from build123d import *

# Parameters (mm, degrees)
SKETCH1_W                  = 177.8
SKETCH1_H                  = 25.4
BOSS_EXTRUDE1_DEPTH        = 9.525
F_1_2_0_5_DIAMETER_HOLE1_D = 12.7
SKETCH6_W                  = 17.78
SKETCH6_H                  = 25.4
CUT_EXTRUDE2_DEPTH         = 180.857514786


with BuildPart() as part:
    # Sketch1 → Boss-Extrude1 (new body)
    with BuildSketch(Plane.XY):
        with Locations((88.9, 12.7)):
            Rectangle(SKETCH1_W, SKETCH1_H)
    extrude(amount=BOSS_EXTRUDE1_DEPTH)

    # 1/2 (0.5) Diameter Hole1 (through all)
    with Locations(Plane.XY.offset(9.525)):
        with Locations((12.7, 12.7), (147.32, 12.7)):
            Hole(F_1_2_0_5_DIAMETER_HOLE1_D / 2)

    # Sketch6 → Cut-Extrude2 (cut, through all)
    with BuildSketch(Plane.XY.offset(9.525)):
        with Locations((168.91, 12.7)):
            Rectangle(SKETCH6_W, SKETCH6_H)
    extrude(amount=-CUT_EXTRUDE2_DEPTH, mode=Mode.SUBTRACT)


solid = part.part
The listing builds one solid part. Answer for the finished solid, in the listing's coordinates (mm). Give positions to 0.01 mm unless a question says otherwise; leave off trailing zeros. Loops run counter-clockwise (first coordinate to the right, second up) from the corner with the lowest first, then second, coordinate; pieces in that order, holes last. Notation, with made-up numbers: (52, 13) - (70, 13) arc R34 ccw to (70, 45) - close; hole circle Ø9 at (87, 18). An arc over 180 degrees is marked (long way). Write each question's results on one line, items separated by ' | '.
1. A flat-ended cylindrical pin translates along its axis: P1, Ø3, axis at x = 72, z = 2.5, coming from the -Y side. Find the tip coordinate at first contact, or state that the pin passes through.
Resolved:
P1: stops at y = 0
2. Find section C-C, the plane z = 1.5. Write down the section's boundary in (x, y).
Resolved:
outline: (0, 0) - (160.02, 0) - (160.02, 25.4) - (0, 25.4) - close; hole circle Ø12.7 at (12.7, 12.7); hole circle Ø12.7 at (147.32, 12.7)
3. Find section B-B, the plane x = 147.32. Write down the section's boundary in (y, z) (3 decimals), then the cut area to 3 significant figures.
Resolved:
outline: (0, 0) - (6.35, 0) - (6.35, 9.525) - (0, 9.525) - close; (19.05, 0) - (25.4, 0) - (25.4, 9.525) - (19.05, 9.525) - close | area: 121 mm^2
4. Consider probe 1 along Y at (x, z) = (12.7, 4); probe 2 along X at (y, z) = (12, 8.75); probe 3 along X at (y, z) = (14.25, 6.5). Determine where each line is inside the solid, lowest interval first. Write a range as from..to.
Resolved:
probe 1: y = 0..6.35, 19.05..25.4 | probe 2: x = 0..6.39, 19.01..141.01, 153.63..160.02 | probe 3: x = 0..6.54, 18.86..141.16, 153.48..160.02
5. Find section A-A, the plane y = 12.7. Write down the section's boundary in (x, z) (3 decimals).
Resolved:
outline: (0, 0) - (6.35, 0) - (6.35, 9.525) - (0, 9.525) - close; (19.05, 0) - (140.97, 0) - (140.97, 9.525) - (19.05, 9.525) - close; (153.67, 0) - (160.02, 0) - (160.02, 9.525) - (153.67, 9.525) - close
6. For a pull along Y with two mould halves and no side action, classify faces 1 (the face through (141.263, 14.607, 4.696)), 2 (the face through (79, 0, 5)), 3 (the face through (0, 13, 5)), 4 (the face through (9.286, 18.054, 4.696)) as +Y half, -Y half, draft (parallel to the pull), parting line (faces both ways), or undercut.
Resolved:
face 1: undercut | face 2: -Y half | face 3: draft | face 4: undercut
